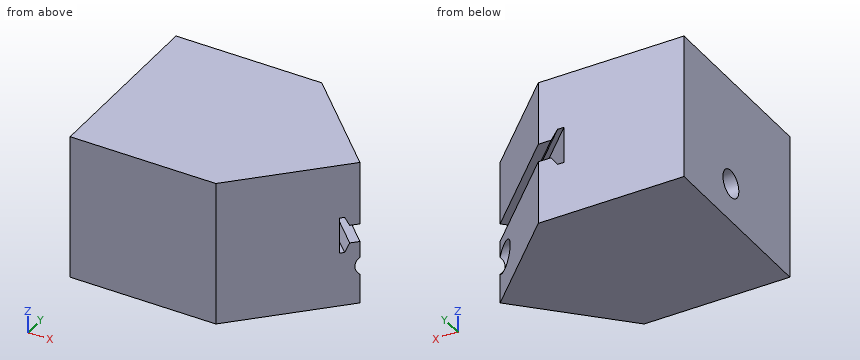
```python
from build123d import *

# Parameters (mm, degrees)
EXTRUDE_1_DEPTH          = 40
SKETCH_2_R               = 7.5
CUT_EXTRUDE_1_DEPTH      = 154.948043183
CUT_EXTRUDE_2_DEPTH      = 141.356688476
CUT_EXTRUDE_2_DEPTH_BACK = 141.356688476
CUT_EXTRUDE_3_DEPTH      = 169.819430161
CUT_EXTRUDE_3_DEPTH_BACK = 169.819430161
SKETCH_4_W               = 39.056064152
SKETCH_4_H               = 128.107121435


with BuildPart() as part:
    # 草图1 → 凸台-拉伸1 (new, symmetric)
    with BuildSketch(Plane.XY):
        Polygon((-140, 50), (-140, -50), (-50, -50), (0, 0), (-50, 50), align=None)
    extrude(amount=EXTRUDE_1_DEPTH, both=True)

    # 草图2 → 切除-拉伸1 (cut, through all)
    with BuildSketch(Plane.ZY.offset(140)):
        with Locations((-18.807269804, 5.733234466)):
            Circle(SKETCH_2_R)
    extrude(amount=-CUT_EXTRUDE_1_DEPTH, mode=Mode.SUBTRACT)

    # 草图3 → 切除-拉伸2 (cut, two sides: drawn at the far end of the back side and taken through both)
    with BuildSketch(Plane(origin=(-50, 50, 0), x_dir=(0, 0, -1), z_dir=(0.7071067811865509, -0.7071067811865441, 0)).offset(-CUT_EXTRUDE_2_DEPTH_BACK)):
        Polygon((5, 5), (-5, 5), (-5, -5), (-10, -7.5), (-10, -10), (10, -10), (10, -7.5), (5, -5), align=None)
    extrude(amount=CUT_EXTRUDE_2_DEPTH + CUT_EXTRUDE_2_DEPTH_BACK, mode=Mode.SUBTRACT)

    # 草图4 → 切除-拉伸3 (cut, two sides: drawn at the far end of the back side and taken through both)
    with BuildSketch(Plane.XY.offset(40).offset(-CUT_EXTRUDE_3_DEPTH_BACK)):
        with Locations((-149.528032076, -5.637932913)):
            Rectangle(SKETCH_4_W, SKETCH_4_H)
    extrude(amount=CUT_EXTRUDE_3_DEPTH + CUT_EXTRUDE_3_DEPTH_BACK, mode=Mode.SUBTRACT)


solid = part.part
```
Model file for the job. Use its own axes, mm. Coordinates: 2 decimals unless noted, no trailing zeros. Loops run counter-clockwise (first coordinate to the right, second up) from the corner with the lowest first, then second, coordinate; pieces in that order, holes last. Notation, with made-up numbers: (32, 29) - (65, 29) arc R14 cw to (65, 36) - close; hole circle Ø3 at (19.5, -4.5). An arc over 180 degrees is marked (long way). Write item = value, one per line. Start each with the question number.
Item 1: Wall check: probe 1 along Z at (x, y) = (-40, 5.5); probe 2 along X at (y, z) = (6.5, -9); probe 3 along Y at (x, z) = (-118, -13.5). Give the ranges that are in metal, low to high. Write a range as [from, to].
Item 2: Saw through at C-C, the plane x = -32.5. List the corners of the cut face in (y, z).
Item 3: Saw through at A-A, the plane y = 2.5. List the corners of the cut face in (x, z).
Item 4: Saw through at B-B, the plane z = 8. List the corners of the cut face in (x, y).
Item 5: Saw through at D-D, the plane y = 28.5. List the corners of the cut face in (x, z).
Item 6: Drop flat-ended pins along their axis: pin 1 Ø2 at (y, z) = (18, -27.5) entering from +X; pin 2 Ø10 at (y, z) = (-12, 17.5) entering from +X; pin 3 Ø24 at (y, z) = (5.73, -18.81) entering from +X. Give the stop position or say it passes through.
Answers:
q1.probe_1 = [-40, -26.3], [-11.31, 40]
q1.probe_2 = [-130, -20.64], [-16.4, -6.5]
q1.probe_3 = [-50, 0.43], [11.03, 50]
q2.outline = (-32.5, -40) - (32.5, -40) - (32.5, -5) - (25.43, -5) - (21.89, -10) - (18.36, -10) - (18.36, 10) - (21.89, 10) - (25.43, 5) - (32.5, 5) - (32.5, 40) - (-32.5, 40) - close; hole circle Ø15 at (5.73, -18.81)
q3.outline = (-130, -40) - (-2.5, -40) - (-2.5, -25.57) - (-130, -25.57) - close; (-130, -12.04) - (-2.5, -12.04) - (-2.5, -5) - (-9.57, -5) - (-13.11, -10) - (-16.64, -10) - (-16.64, 10) - (-13.11, 10) - (-9.57, 5) - (-2.5, 5) - (-2.5, 40) - (-130, 40) - close
q4.outline = (-130, -50) - (-50, -50) - (-7.07, -7.07) - (-64.14, 50) - (-130, 50) - close; (-59.19, 50) - (-4.6, -4.6) - (0, 0) - (-50, 50) - close
q5.outline = (-130, -40) - (-28.5, -40) - (-28.5, -5) - (-35.57, -5) - (-39.11, -10) - (-42.64, -10) - (-42.64, 10) - (-39.11, 10) - (-35.57, 5) - (-28.5, 5) - (-28.5, 40) - (-130, 40) - close
q6.pin_1 = -17
q6.pin_2 = -7
q6.pin_3 = 0
